Model file for the job. Use its own axes, mm. Round coordinates to 2 decimals unless told otherwise and drop trailing zeros. Order: outer loops, then holes, each group sorted by start corner. A loop starts at its lowest first (then second) coordinate and runs counter-clockwise, first axis right, second up. Notation, with made-up numbers: M 56,84.5 L 96,84.5 A24 cw 96,101.5 Z; hole C 23,-13.75 d7. An arc over 180 degrees is marked long. Return JSON: item names as keys, results as strings. Group by question number.
Item 1: Slice it at A-A on z = 44.5. Write the cut outline in (x, y), then the cut area to 3 significant figures.
Item 2: Slice it at B-B on z = 28. Write the cut outline in (x, y).
Item 3: Probe line 1 along Z through (x, y) = (-13, -0.5); line 2 along X through (y, z) = (-1, -3); line 3 along Y through (x, z) = (-3.5, 32). List the from-to ranges inside material, lowest first.
Item 4: Pin check, flat tips, straight feed: pin 1 Ø12 at (y, z) = (-14.5, 41.5) entering from -X; pin 2 Ø1.5 at (x, y) = (-2, -16) entering from -Z; pin 3 Ø8 at (x, y) = (15, 15) entering from +Z; pin 4 Ø4 at (x, y) = (-10.5, -6.5) entering from -Z. Stop position of each tip, or through.
Item 5: Pull direction X, two halves, no side cores. Call faces 1 (the face through (-14.98, 10.73, -1.88)), 2 (the face through (6.88, -8.71, 15.105)), 3 (the face through (1.3, -0.31, 6.11)): pulls with the +X half, pulls with the -X half, needs draft (parallel to the pull), parting line crosses it, or undercut.
from build123d import *

# Parameters (mm, degrees)
F3_DEPTH      = 11.001
F3_DEPTH_BACK = 11.001
F5_DEPTH      = 4
F6_R          = 3
F7_R          = 2.69


with BuildPart() as f1:
    # F0 (on Front) → F1 (revolve)
    with BuildSketch(Plane.XZ):
        Polygon((-4.066010414, 66), (-11, 0), (0, 0), (0, 66), align=None)
    revolve(axis=Axis((0, 0, 33), (0, 0, -1)))

    # F2 (on Front) → F3 (cut, two sides)
    with BuildSketch(Plane.XZ) as f3_sk:
        Polygon((40.7802015543, 39.7115387022), (-13.9303933829, 0), (40.7802015543, 0), align=None)
    extrude(amount=-F3_DEPTH, mode=Mode.SUBTRACT)
    extrude(f3_sk.sketch, amount=F3_DEPTH_BACK, mode=Mode.SUBTRACT)

    # F4 (on face) → F5 (join)
    with BuildSketch(Plane(origin=(-4.8068030747, 0, 6.6223335725), x_dir=(0.8092844528, 0, 0.5874169511), z_dir=(0.5874169511, 0, -0.8092844528))):
        Polygon((-7.7040281941, -22), (17.6993836503, -22), (30.4010895725, 0), (17.6993836503, 22), (-7.7040281941, 22), (-20.4057341162, 0), align=None)
    extrude(amount=F5_DEPTH)

    # F6
    f6_edges = [f1.edges().sort_by_distance(p)[0] for p in [
        (-0.76226, 22, 9.558054),
        (14.65668, 11, 20.74985),
        (14.65668, -11, 20.74985),
        (-0.76226, -22, 9.558054),
        (-16.1812, -11, -1.633742),
        (-16.1812, 11, -1.633742),
    ]]
    fillet(f6_edges, radius=F6_R)

    # F7
    f7_edges = [f1.edges().sort_by_distance(p)[0] for p in [
        (4.06601, 0, 66),
    ]]
    fillet(f7_edges, radius=F7_R)


solid = f1.part
Output values:
{
 "1": {"outline": "C 0,0 d12.65", "area": "126 mm²"},
 "2": {"outline": "C 0,0 d16.12"},
 "3": {"line 1": "-4.27 to 0.68", "line 2": "-18.06 to -11.25", "line 3": "-6.79 to 6.79"},
 "4": {"pin 1": "through", "pin 2": "z = 3.17", "pin 3": "z = 19.42", "pin 4": "z = -3.9"},
 "5": {"face 1": "pulls with the -X half", "face 2": "undercut", "face 3": "pulls with the +X half"}
}
